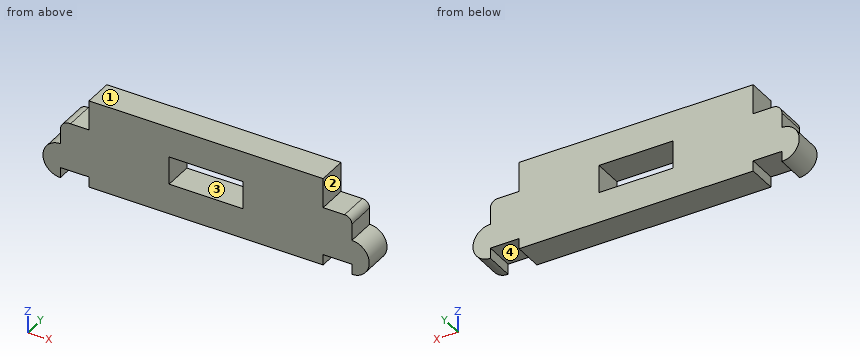
from build123d import *

# Parameters (mm, degrees)
SKETCH2_W           = 7.98583157
SKETCH2_H           = 3.000090293
BOSS_EXTRUDE1_DEPTH = 3.175


with BuildPart() as part:
    # Sketch2 → Boss-Extrude1 (new body)
    with BuildSketch(Plane(origin=(0, 0, 0), x_dir=(1, 0, 0), z_dir=(0, 1, 0))):
        with BuildLine():
            Line((12.625998491, -1.744524944), (12.625998491, -4.950391186))
            Line((12.625998491, -4.950391186), (-12.629130241, -4.950391186))
            Line((-12.629130241, -4.950391186), (-12.629130241, -1.744524944))
            Line((-12.629130241, -1.744524944), (-14.623097356, -1.744524944))
            ThreePointArc((-14.623097356, -1.744524944), (-15.39182083, -1.504361603), (-15.722173536, -0.769867695))
            Line((-15.722173536, -0.769867695), (-15.722173536, 0.826844293))
            ThreePointArc((-15.722173536, 0.826844293), (-17.599363905, 2.704034662), (-15.722173536, 4.581225032))
            Line((-15.722173536, 4.581225032), (-15.722173536, 3.471753772))
            Line((-15.722173536, 3.471753772), (-12.631299313, 3.460874113))
            Line((-12.631299313, 3.460874113), (-12.631299313, 4.586967616))
            Line((-12.631299313, 4.586967616), (12.625998491, 4.586967616))
            Line((12.625998491, 4.586967616), (12.625998491, 3.460874113))
            Line((12.625998491, 3.460874113), (15.720511393, 3.460874113))
            Line((15.720511393, 3.460874113), (15.720511393, 4.581225031))
            ThreePointArc((15.720511393, 4.581225031), (17.597858023, 2.703878401), (15.720511393, 0.826531771))
            Line((15.720511393, 0.826531771), (15.720511393, -0.972713755))
            ThreePointArc((15.720511393, -0.972713755), (15.488390746, -1.524540285), (14.931614971, -1.744524944))
            Line((14.931614971, -1.744524944), (12.625998491, -1.744524944))
        make_face()
        with Locations((2.437e-06, -0.181702019)):
            Rectangle(SKETCH2_W, SKETCH2_H, mode=Mode.SUBTRACT)
    extrude(amount=BOSS_EXTRUDE1_DEPTH)


solid = part.part
Read the model definition and answer for the solid it produces. Units are mm, in the model's axes. Face numbers are marked on the shaded views. A direction names the side the tool comes from. Give positions to 0.01 mm unless a question says otherwise; leave off trailing zeros. Write each loop counter-clockwise with the first axis right and the second up, starting at its lowest first coordinate (ties: lowest second). Pieces come first, ordered by that corner, then holes. Notation, with made-up numbers: (59, 9) - (100, 9) arc R24 cw to (100, 39) - close; hole circle Ø10 at (-17, 64). An arc over 180 degrees is marked (long way). Use CSV: the item, a comma, the result in double quotes. Start each with the question number.
Item 1: Consider line 1 (X direction, y = 1.5, z = 0.25); line 2 (X direction, y = 1.7, z = -3.75); line 3 (Z direction, x = 2, y = 3). Determine where each line is inside the solid, lowest interval first.
Item 2: The part is cut by section D-D, the plane z = 3.75. Give the vertices of the cut face in (x, y) (3 decimals).
Item 3: The part is cut by section B-B, the plane z = -0.5. Give the vertices of the cut face in (x, y) (3 decimals).
Item 4: The part is cut by section C-C, the plane x = -2.5. Give the vertices of the cut face in (y, z) (3 decimals), and give its area (3 significant figures).
Item 5: For the marked faces 1, 2, 3 and 4, determine the directions among +Z, -Z, +X, -X, +Y, -Y from which every point of the face is accessible in a straight line to the end or side of a thin tool.
Item 6: The part is cut by section A-A, the plane y = 0.85. Give the vertices of the cut face in (x, z), and give its area (3 significant figures).
Item 7: Flat-ended cylindrical pins translate along their axes: P1, Ø1, axis at y = 1.5, z = 3, coming from the -X side; P2, Ø1, axis at y = 1, z = 1.5, coming from the +X side; P3, Ø1.2, axis at y = 1, z = -4, coming from the +X side. Find the tip coordinate at first contact, or state that the pin passes through.
Taken from the geometry:
1,line 1,"-15.72 to -3.99, 3.99 to 15.72"
1,line 2,"-17.28 to -15.72, -12.63 to 12.63, 15.72 to 17.28"
1,line 3,"-4.59 to -1.32, 1.68 to 4.95"
2,outline,"(-12.629, 0) - (12.626, 0) - (12.626, 3.175) - (-12.629, 3.175) - close"
3,outline,"(-15.722, 0) - (-3.993, 0) - (-3.993, 3.175) - (-15.722, 3.175) - close; (3.993, 0) - (15.721, 0) - (15.721, 3.175) - (3.993, 3.175) - close"
4,outline,"(0, -4.587) - (3.175, -4.587) - (3.175, -1.318) - (0, -1.318) - close; (0, 1.682) - (3.175, 1.682) - (3.175, 4.95) - (0, 4.95) - close"
4,area,"20.8 mm2"
5,face 1,"+Z, +X, -X, +Y, -Y"
5,face 2,"+Z, +X, +Y, -Y"
5,face 3,"+Y, -Y"
5,face 4,"-Z, +Y, -Y"
6,outline,"(-15.72, -4.58) - (-15.72, -3.47) - (-12.63, -3.46) - (-12.63, -4.59) - (12.63, -4.59) - (12.63, -3.46) - (15.72, -3.46) - (15.72, -4.58) arc R1.88 ccw to (15.72, -0.83) - (15.72, 0.97) arc R0.77 ccw to (14.93, 1.74) - (12.63, 1.74) - (12.63, 4.95) - (-12.63, 4.95) - (-12.63, 1.74) - (-14.62, 1.74) arc R0.98 ccw to (-15.72, 0.77) - (-15.72, -0.83) arc R1.88 ccw to start; hole (-3.99, -1.32) - (3.99, -1.32) - (3.99, 1.68) - (-3.99, 1.68) - close"
6,area,"260 mm2"
7,P1,"x = -12.63"
7,P2,"x = 15.72"
7,P3,"x = 17.46"
